```python
from build123d import *

# Parameters (mm, degrees)
SKETCH1_W           = 110
SKETCH1_H           = 50
SKETCH1_R           = 10
BOSS_EXTRUDE1_DEPTH = 3.175
FILLET1_R           = 5


with BuildPart() as part:
    # Sketch1 → Boss-Extrude1 (new, symmetric)
    with BuildSketch(Plane(origin=(0, 0, 0), x_dir=(0, 0, -1), z_dir=(1, 0, 0))):
        with Locations((-25, 0)):
            Rectangle(SKETCH1_W, SKETCH1_H)
        Circle(SKETCH1_R, mode=Mode.SUBTRACT)
    extrude(amount=BOSS_EXTRUDE1_DEPTH, both=True)

    # Fillet1
    fillet1_edges = [part.edges().sort_by_distance(p)[0] for p in [
        (0, -25, -30),
        (0, 25, -30),
    ]]
    fillet(fillet1_edges, radius=FILLET1_R)


solid = part.part
```
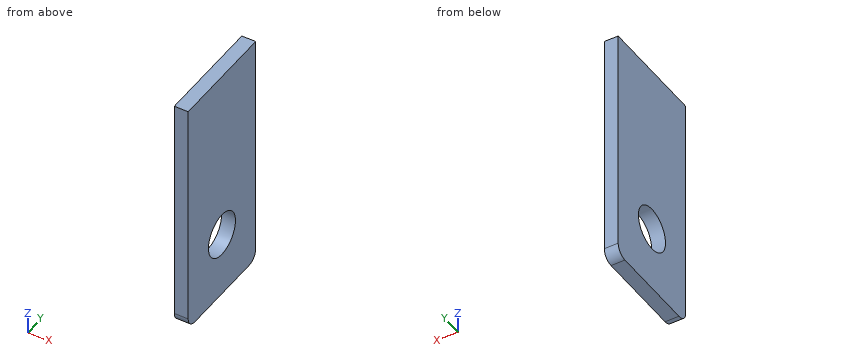
CAD build for the part. Positions are in the model's coordinates, mm. Coordinates: 2 decimals unless noted, no trailing zeros. Order: outer loops, then holes, each group sorted by start corner. A loop starts at its lowest first (then second) coordinate and runs counter-clockwise, first axis right, second up.
(1) Drill centre lines: L1, parallel to Y at x = -1.5, z = 0; L2, parallel to Y at x = 0.75, z = 3; L3, parallel to Z at x = 1.75, y = -4. Where is each one in solid material? Low to high.
Solution:
L1: y = -25 to -10, 10 to 25
L2: y = -25 to -9.54, 9.54 to 25
L3: z = -30 to -9.17, 9.17 to 80
(2) Saw through at B-B, the plane x = 0.5. Write the cut outline in (y, z).
Solution:
outline: (-25, -25) arc R5 ccw to (-20, -30) - (20, -30) arc R5 ccw to (25, -25) - (25, 80) - (-25, 80) - close; hole circle Ø20 at (0, 0)
(3) Saw through at A-A, the plane y = 0. Write the cut outline in (x, z) (3 decimals), and give its area (4 significant figures).
Solution:
outline: (-3.175, -30) - (3.175, -30) - (3.175, -10) - (-3.175, -10) - close; (-3.175, 10) - (3.175, 10) - (3.175, 80) - (-3.175, 80) - close
area: 571.5 mm2
(4) Saw through at C-C, the plane z = 0. Write the cut outline in (x, y) (3 decimals), and give its area (4 significant figures).
Solution:
outline: (-3.175, -25) - (3.175, -25) - (3.175, -10) - (-3.175, -10) - close; (-3.175, 10) - (3.175, 10) - (3.175, 25) - (-3.175, 25) - close
area: 190.5 mm2
